The listing builds one solid part. Answer for the finished solid, in the listing's coordinates (mm). Face numbers are marked on the shaded views. A direction names the side the tool comes from. Coordinates: 2 decimals unless noted, no trailing zeros. Loops run counter-clockwise (first coordinate to the right, second up) from the corner with the lowest first, then second, coordinate; pieces in that order, holes last. Notation, with made-up numbers: M 2,84.5 L 26,84.5 A29 ccw 26,111.5 Z; hole C 38.25,39 d7. An arc over 180 degrees is marked long. Answer as a JSON object with one key per item and string values. Group by question number.
1. Straight lines are drawn through the part: L1, parallel to Z at x = 18.5, y = 34.5; L2, parallel to Z at x = 37.7, y = -44.35. For each, find the intervals that lie inside material, in ascending order.
2. A cutting plane is placed at B-B on y = 0. Give the vertices of the cut face in (x, z) (3 decimals), and give its area (3 significant figures).
3. A cutting plane is placed at A-A on x = 37.7. Give the vertices of the cut face in (y, z), and give its area (3 significant figures).
4. Given pin 1 (8 mm diameter, centred on y = 19.5, z = -20, fed in from +X), flat-ended and moving along its own axis, determine where the tip first touches the part or whether it passes through.
5. A cutting plane is placed at D-D on x = 15.5. Give the vertices of the cut face in (y, z).
6. Determine the mould class of the marked faces 3, 4 and 5 for opening direction Z: released by +Z, released by -Z, zero draft, split by the parting line, or undercut.
7. For the marked faces 1 and 2, determine the directions among +Z, -Z, +X, -X, +Y, -Y from which every point of the face is accessible in a straight line to the end or side of a thin tool.
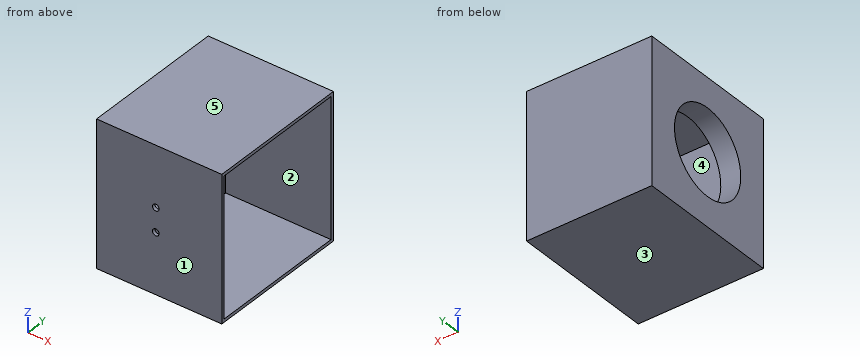
from build123d import *

# Parameters (mm, degrees)
SKETCH1_W                       = 92
SKETCH1_H                       = 92
SKETCH1_W_2                     = 88
SKETCH1_H_2                     = 88
SKETCH1_R                       = 27.305
BOSS_EXTRUDE1_DEPTH             = 12.7
SKETCH2_W                       = 92
SKETCH2_H                       = 92
SKETCH2_W_2                     = 88
SKETCH2_H_2                     = 88
BOSS_EXTRUDE2_DEPTH             = 67
F_19_0_166_DIAMETER_HOLE1_D     = 4.2164
F_19_0_166_DIAMETER_HOLE1_DEPTH = 2


with BuildPart() as part:
    # Sketch1 → Boss-Extrude1 (new body)
    # profile 1 of 2: a face of its own
    with BuildSketch(Plane(origin=(0, 0, 0), x_dir=(0, 0, -1), z_dir=(1, 0, 0))):
        Rectangle(SKETCH1_W, SKETCH1_H)
        Rectangle(SKETCH1_W_2, SKETCH1_H_2, mode=Mode.SUBTRACT)
    # profile 2 of 2: a face of its own
    with BuildSketch(Plane(origin=(0, 0, 0), x_dir=(0, 0, -1), z_dir=(1, 0, 0))):
        Rectangle(SKETCH1_W_2, SKETCH1_H_2)
        Circle(SKETCH1_R, mode=Mode.SUBTRACT)
    extrude(amount=BOSS_EXTRUDE1_DEPTH)

    # Sketch2 → Boss-Extrude2 (add)
    with BuildSketch(Plane(origin=(12.7, 0, 0), x_dir=(0, 0, -1), z_dir=(1, 0, 0))):
        Rectangle(SKETCH2_W, SKETCH2_H)
        Rectangle(SKETCH2_W_2, SKETCH2_H_2, mode=Mode.SUBTRACT)
    extrude(amount=BOSS_EXTRUDE2_DEPTH)

    # #19 (0.166) Diameter Hole1
    with Locations(Plane(origin=(0, -46, 0), x_dir=(-1, 0, 0), z_dir=(0, -1, 0))):
        with Locations((-37.7, 7.62), (-37.7, -7.62), (17.600686592, 72.613770274), (-57.973181852, -74.350642439), (-79.7, -100.115693871), (-40.410274663, -84.366152369)):
            Hole(F_19_0_166_DIAMETER_HOLE1_D / 2, depth=F_19_0_166_DIAMETER_HOLE1_DEPTH)


solid = part.part
From the geometry:
{
 "1": {"L1": "z = -46 to -44, 44 to 46", "L2": "z = -46 to -9.73, -5.51 to 5.51, 9.73 to 46"},
 "2": {"outline": "M 0,-46 L 79.7,-46 L 79.7,-44 L 12.7,-44 L 12.7,-27.305 L 0,-27.305 Z; M 0,27.305 L 12.7,27.305 L 12.7,44 L 79.7,44 L 79.7,46 L 0,46 Z", "area": "743 mm²"},
 "3": {"outline": "M -46,-46 L 46,-46 L 46,46 L -46,46 L -46,9.73 L -44,9.73 L -44,44 L 44,44 L 44,-44 L -44,-44 L -44,-9.73 L -46,-9.73 Z; M -46,-5.51 L -44,-5.51 L -44,5.51 L -46,5.51 Z", "area": "703 mm²"},
 "4": {"pin 1": "stops at x = 12.7"},
 "5": {"outline": "M -46,-46 L 46,-46 L 46,46 L -46,46 Z; hole M -44,-44 L 44,-44 L 44,44 L -44,44 Z"},
 "6": {"face 3": "released by -Z", "face 4": "undercut", "face 5": "released by +Z"},
 "7": {"face 1": "+Z, -Z, +X, -X, -Y", "face 2": "+X"}
}
